Verification items for this drawing (mm, ordinates from the low corner). A direction names the side the tool comes from. Coordinates: 2 decimals unless noted, no trailing zeros. Write each loop counter-clockwise with the first axis right and the second up, starting at its lowest first coordinate (ties: lowest second). Pieces come first, ordered by that corner, then holes. Notation, with made-up numbers: M 89.5,37 L 101.5,37 A28 ccw 101.5,73 Z; hole C 46.5,72.5 d3. An arc over 180 degrees is marked long. Put each result on its own line as item: value. Start each with the question number.
1) Cross-section at D-D on y = 5.5. Record the cut outline in (x, z), plus the area to 3 significant figures.
2) Mould release check, pull along Z, two halves, no side actions. Record for the marked faces 4, 5, 6 and 7: released by +Z, released by -Z, zero draft, split by the parting line, or undercut.
3) Gauge pin test, flat ends, axial feed: pin 1 (1.5 mm diameter, centred on x = 10.5, y = 2.5, fed in from +Z); pin 2 (2.5 mm diameter, centred on y = 3.5, z = 5, fed in from -X); pin 3 (2 mm diameter, centred on x = 12, y = 3, fed in from +Z). Record the tip position at first contact, or that the pin passes through.
4) Cross-section at A-A on y = 3. Count the separate pieces of the cut face and the enclosed holes in it, plus the area to 3 significant figures.
5) Scan lines: line 1 along Y through (x, z) = (12, 0.35); line 2 along Z through (x, y) = (10.5, 0.45); line 3 along X through (y, z) = (2.75, 6.5). Record each from-to range of solid material in increasing order.
6) Cross-section at C-C on x = 12.5. Record the cut outline in (y, z).
7) Cross-section at B-B on z = 3.75. Record the cut outline in (x, y), plus the area to 3 significant figures.
8) Set-up check for the marked faces 1, 2 and 3: record each of +Z, -Z, +X, -X, +Y, -Y from which the full face is reachable in a straight line by a thin tool's end or side.
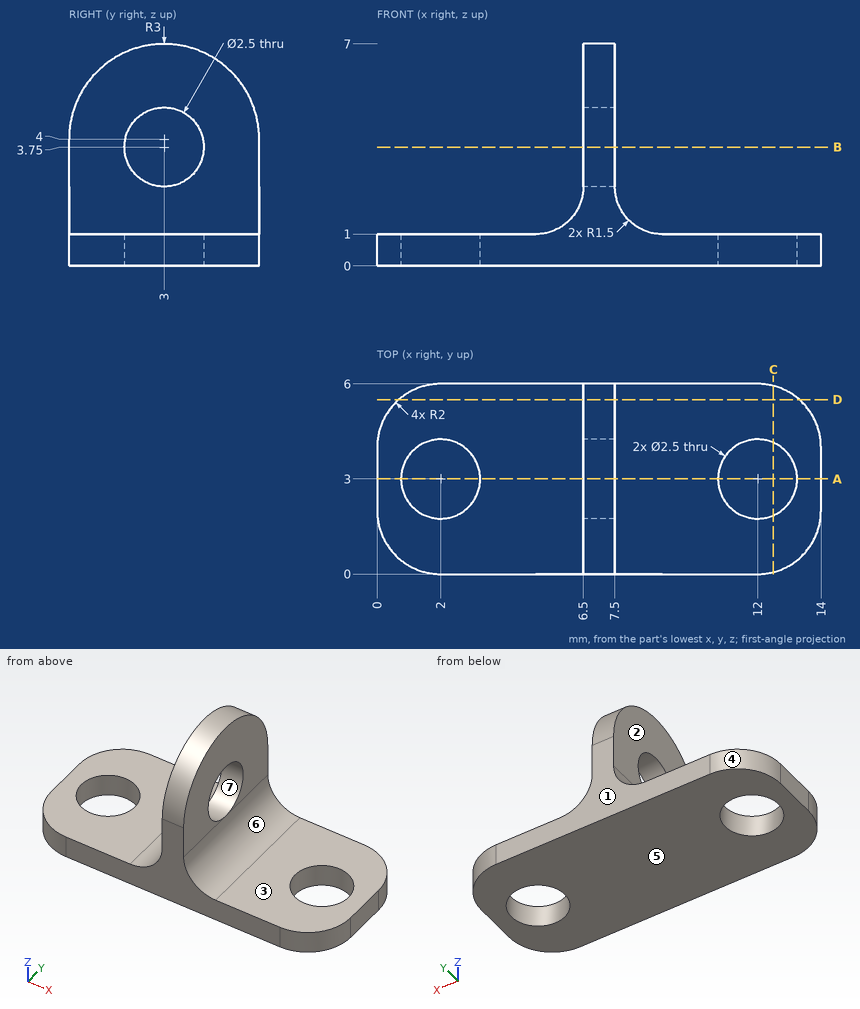
Answer key:
1. outline: M 0.68,0 L 13.32,0 L 13.32,1 L 9,1 A1.5 cw 7.5,2.5 L 7.5,5.66 L 6.5,5.66 L 6.5,2.5 A1.5 cw 5,1 L 0.68,1 Z
1. area: 18.3 mm²
2. face 4: zero draft
2. face 5: released by -Z
2. face 6: released by +Z
2. face 7: undercut
3. pin 1: stops at z = 1
3. pin 2: stops at x = 6.5
3. pin 3: passes through
4. separate pieces: 4
4. enclosed holes: 0
4. area: 13.5 mm²
5. line 1: y = 0 to 1.75, 4.25 to 6
5. line 2: z = 0 to 1
5. line 3: x = 6.5 to 7.5
6. outline: M 0.06,0 L 1.85,0 L 1.85,1 L 0.06,1 Z; M 4.15,0 L 5.94,0 L 5.94,1 L 4.15,1 Z
7. outline: M 6.5,0 L 7.5,0 L 7.5,1.75 L 6.5,1.75 Z; M 6.5,4.25 L 7.5,4.25 L 7.5,6 L 6.5,6 Z
7. area: 3.50 mm²
8. face 1: +Z, -Z, +X, -X, +Y
8. face 2: +Z, -X, +Y, -Y
8. face 3: +Z, +X, +Y, -Y
